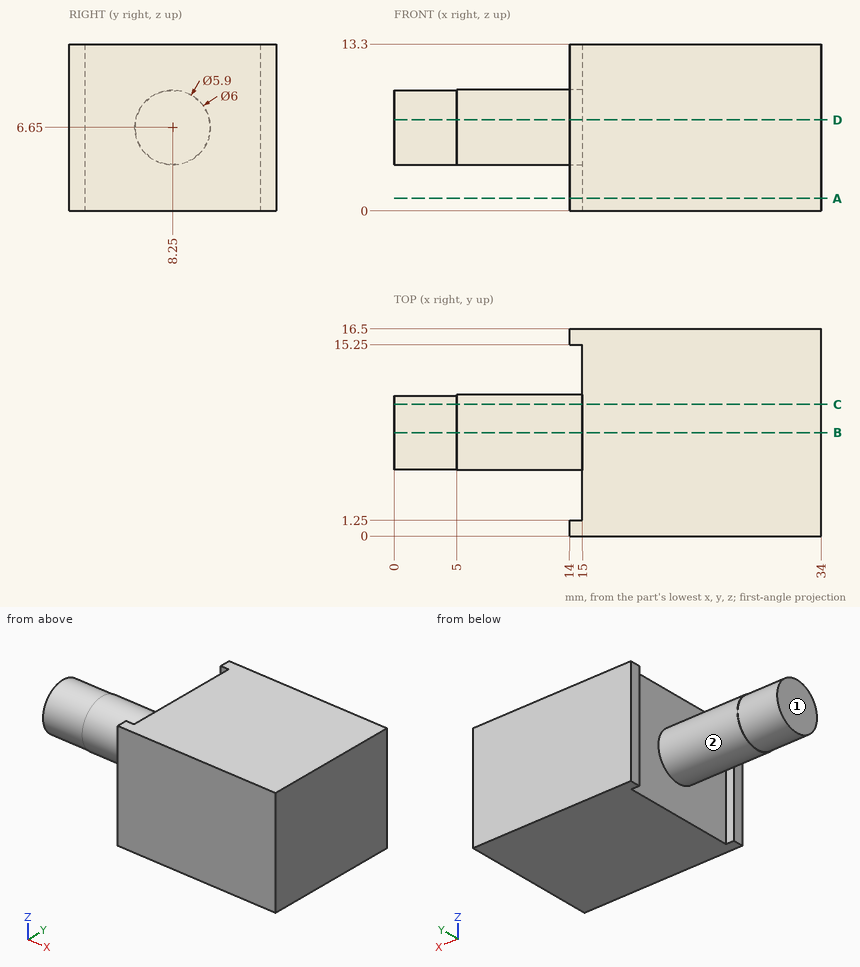
Print and shaded views of the part. All mm, measured from the part's lowest x, y and z. A direction names the side the tool comes from. Round coordinates to 2 decimals unless told otherwise and drop trailing zeros. Write each loop counter-clockwise with the first axis right and the second up, starting at its lowest first coordinate (ties: lowest second). Pieces come first, ordered by that corner, then holes.
Item 1: Cut at B-B, the plane y = 8.25. Give the cut face in (x, z).
Results:
outline: (0, 3.7) - (5, 3.7) - (5, 3.65) - (15, 3.65) - (15, 0) - (34, 0) - (34, 13.3) - (15, 13.3) - (15, 9.65) - (5, 9.65) - (5, 9.6) - (0, 9.6) - close
Item 2: Cut at D-D, the plane z = 7.25. Give the cut face in (x, y).
Results:
outline: (0, 5.36) - (5, 5.36) - (5, 5.31) - (15, 5.31) - (15, 1.25) - (14, 1.25) - (14, 0) - (34, 0) - (34, 16.5) - (14, 16.5) - (14, 15.25) - (15, 15.25) - (15, 11.19) - (5, 11.19) - (5, 11.14) - (0, 11.14) - close
Item 3: Probe L1, parallel to X at y = 8, z = 10.25; L2, parallel to Z at x = 13, y = 10.5; L3, parallel to Y at x = 7, z = 7. List the from-to ranges inside material, lowest first.
Results:
L1: x = 15 to 34
L2: z = 4.67 to 8.63
L3: y = 5.27 to 11.23
Item 4: Cut at A-A, the plane z = 1. Give the cut face in (x, y), plus the area to 3 significant figures.
Results:
outline: (14, 0) - (34, 0) - (34, 16.5) - (14, 16.5) - (14, 15.25) - (15, 15.25) - (15, 1.25) - (14, 1.25) - close
area: 316 mm2
Item 5: Cut at C-C, the plane y = 10.5. Give the cut face in (x, z), plus the area to 3 significant figures.
Results:
outline: (0, 4.74) - (5, 4.74) - (5, 4.67) - (15, 4.67) - (15, 0) - (34, 0) - (34, 13.3) - (15, 13.3) - (15, 8.63) - (5, 8.63) - (5, 8.56) - (0, 8.56) - close
area: 311 mm2
Item 6: Which spindle directions (+Z, -Z, +X, -X, +Y, -Y) get a long thin tool onto all of the face, cutting with end or side? Do the marked faces 1 and 2. Say none if no direction does.
Results:
face 1: +Z, -Z, -X, +Y, -Y
face 2: -X
Item 7: Drop flat-ended pins along their axis: pin 1 Ø5 at (x, z) = (5.5, 10.5) entering from -Y; pin 2 Ø1.5 at (x, y) = (13.5, 9) entering from +Z; pin 3 Ø1 at (y, z) = (16, 6) entering from -X. Give the stop position or say it passes through.
Results:
pin 1: stops at y = 5.57
pin 2: stops at z = 9.65
pin 3: stops at x = 14
